Could you check a few things on this drawing? It's one solid part, dimensions in mm from its lowest x, y, z. A direction names the side the tool comes from. Give positions to 0.01 mm unless a question says otherwise; leave off trailing zeros. Order: outer loops, then holes, each group sorted by start corner. A loop starts at its lowest first (then second) coordinate and runs counter-clockwise, first axis right, second up. Notation, with made-up numbers: (40.25, 71.25) -> (85.25, 71.25) arc R28 cw to (85.25, 94.25) -> close; hole circle Ø4 at (18, 42.5). An arc over 180 degrees is marked (long way). Answer as CSV lines item,"result".
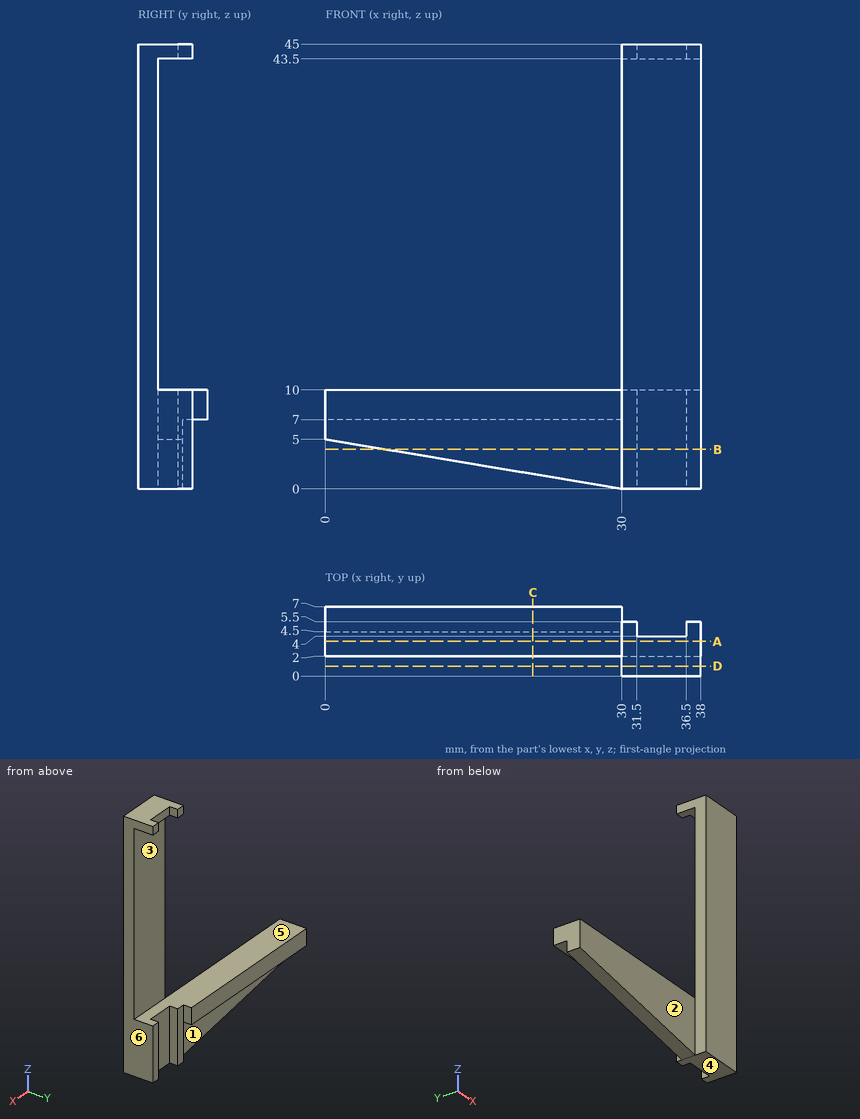
Item 1: Imagine slicing it at A-A, the plane y = 3.5. Please give me the cut outline in (x, z).
Numbers:
outline,"(0, 5) -> (30, 0) -> (38, 0) -> (38, 10) -> (0, 10) -> close; (30, 43.5) -> (38, 43.5) -> (38, 45) -> (30, 45) -> close"
Item 2: We'd pull the mould along Z, two halves only. Please class the marked faces 4, 5 and 6: released by +Z, released by -Z, zero draft, split by the parting line, or undercut.
Numbers:
face 4,"released by -Z"
face 5,"undercut"
face 6,"zero draft"
Item 3: For the marked faces 1, 2 and 3, which set-ups out of +Z, -Z, +X, -X, +Y, -Y let a thin tool reach every point of the face, with its end or its side?
Numbers:
face 1,"-Z, -X, +Y"
face 2,"+Z, -Z, -X, -Y"
face 3,"+X, -X, +Y"
Item 4: Imagine slicing it at B-B, the plane z = 4. Please give me the cut outline in (x, y).
Numbers:
outline,"(6, 2) -> (30, 2) -> (30, 0) -> (38, 0) -> (38, 5.5) -> (36.5, 5.5) -> (36.5, 4) -> (31.5, 4) -> (31.5, 5.5) -> (30, 5.5) -> (30, 4.5) -> (6, 4.5) -> close"
Item 5: Imagine slicing it at C-C, the plane x = 21. Please give me the cut outline in (y, z).
Numbers:
outline,"(2, 1.5) -> (4.5, 1.5) -> (4.5, 7) -> (7, 7) -> (7, 10) -> (2, 10) -> close"
Item 6: Imagine slicing it at D-D, the plane y = 1. Please give me the cut outline in (x, z), then the cut area to 3 significant figures.
Numbers:
outline,"(30, 0) -> (38, 0) -> (38, 45) -> (30, 45) -> close"
area,"360 mm²"
Item 7: Please list where these lines run through material, in increasing order: line 1 along Z through (x, y) = (6, 6.75); line 2 along Z through (x, y) = (30.5, 3.5); line 3 along Y through (x, z) = (8, 9).
Numbers:
line 1,"z = 7 to 10"
line 2,"z = 0 to 10, 43.5 to 45"
line 3,"y = 2 to 7"
Item 8: For pin 1 (0.8 mm diameter, centred on y = 6.5, z = 8.5, fed in from +X); pin 2 (0.8 mm diameter, centred on x = 37, z = 5.5, fed in from +Y); pin 3 (3 mm diameter, centred on x = 13, y = 5.5, fed in from -Z), each with a flat end and sliding along its axis, tell me the tip position at first contact or that it passes through.
Numbers:
pin 1,"stops at x = 30"
pin 2,"stops at y = 5.5"
pin 3,"stops at z = 2.65"
